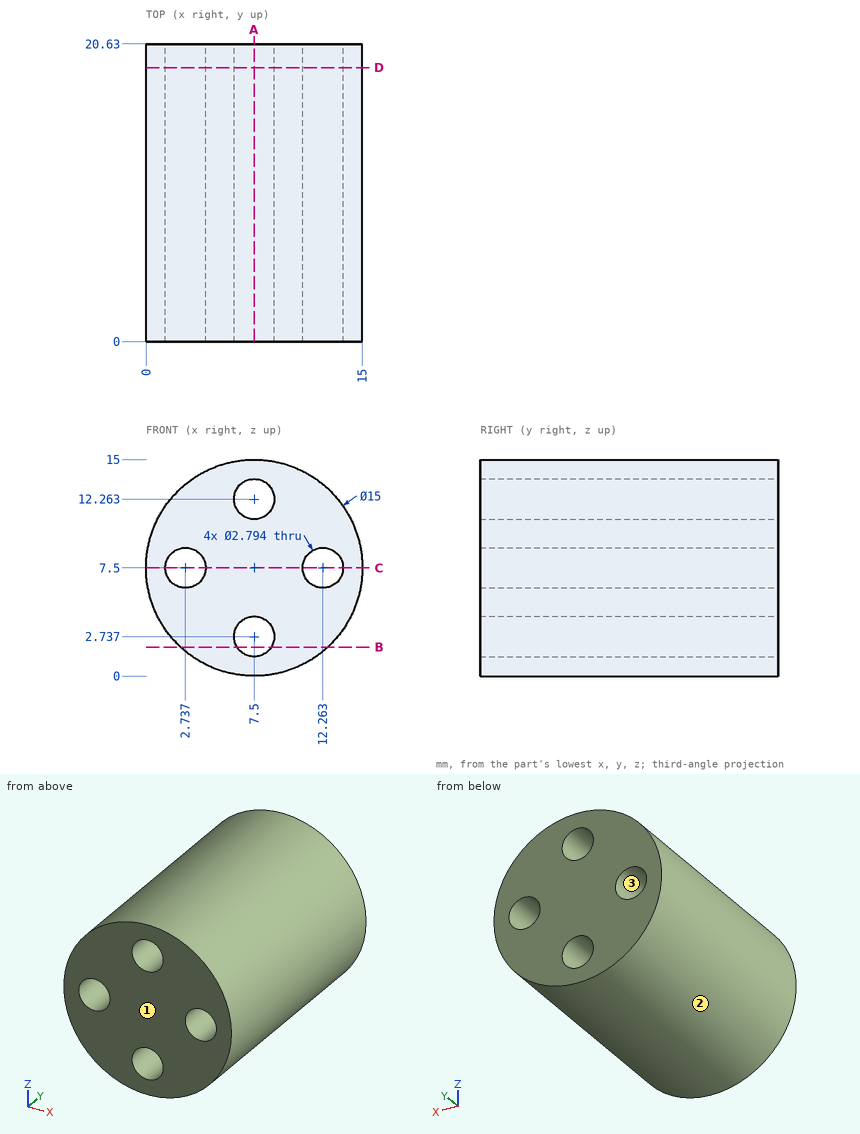
Job drawing, mm, ordinate dimensions from the low corner. One solid piece. Coordinates: 2 decimals unless noted, no trailing zeros. Write each loop counter-clockwise with the first axis right and the second up, starting at its lowest first coordinate (ties: lowest second). Pieces come first, ordered by that corner, then holes. Notation, with made-up numbers: (34, 33) - (65, 33) arc R23 cw to (65, 47) - close; hole circle Ø6 at (12.5, 36.25). An arc over 180 degrees is marked (long way). Use a Markdown table: item, result. Add a question column.
Item 1: Mould opens along X. For the marked faces 1, 2 and 3 say: pulls with the +X half, pulls with the -X half, needs draft (parallel to the pull), parting line crosses it, or undercut.
Item 2: Flat gauge pins, fed straight in: pin 1 (1.7 mm diameter, centred on x = 2.74, z = 7.5, fed in from +Y); pin 2 (1 mm diameter, centred on y = 7, z = 9, fed in from -X). Where does each tip first touch, or does it go through?
Item 3: Band-saw the part on C-C, the plane z = 7.5. Give the cut face in (x, y) (1 decimal), and give its area (3 significant figures).
Item 4: Drill centre lines: L1, parallel to X at y = 9.25, z = 7.5 (1 decimal); L2, parallel to X at y = 14, z = 6.75 (1 decimal). Where is each one in solid material? Low to high. Write a range as from..to.
Item 5: Band-saw the part on B-B, the plane z = 2. Give the cut face in (x, y).
Item 6: Band-saw the part on A-A, the plane x = 7.5. Give the cut face in (y, z) (1 decimal).
Item 7: Band-saw the part on D-D, the plane y = 19. Give the cut face in (x, z) (1 decimal).
Numbers:
| question | item | result |
|---|---|---|
| 1 | face 1 | needs draft |
| 1 | face 2 | parting line crosses it |
| 1 | face 3 | undercut |
| 2 | pin 1 | through |
| 2 | pin 2 | x = 0.07 |
| 3 | outline | (0, 0) - (1.3, 0) - (1.3, 20.6) - (0, 20.6) - close; (4.1, 0) - (10.9, 0) - (10.9, 20.6) - (4.1, 20.6) - close; (13.7, 0) - (15, 0) - (15, 20.6) - (13.7, 20.6) - close |
| 3 | area | 194 mm2 |
| 4 | L1 | 0..1.3, 4.1..10.9, 13.7..15 |
| 4 | L2 | 0..1.6, 3.9..11.1, 13.4..15 |
| 5 | outline | (2.4, 0) - (6.31, 0) - (6.31, 20.63) - (2.4, 20.63) - close; (8.69, 0) - (12.6, 0) - (12.6, 20.63) - (8.69, 20.63) - close |
| 6 | outline | (0, 0) - (20.6, 0) - (20.6, 1.3) - (0, 1.3) - close; (0, 4.1) - (20.6, 4.1) - (20.6, 10.9) - (0, 10.9) - close; (0, 13.7) - (20.6, 13.7) - (20.6, 15) - (0, 15) - close |
| 7 | outline | circle Ø15 at (7.5, 7.5); hole circle Ø2.8 at (2.7, 7.5); hole circle Ø2.8 at (7.5, 2.7); hole circle Ø2.8 at (7.5, 12.3); hole circle Ø2.8 at (12.3, 7.5) |
